Job drawing, mm, ordinate dimensions from the low corner. One solid piece. Coordinates: 2 decimals unless noted, no trailing zeros. Loops run counter-clockwise (first coordinate to the right, second up) from the corner with the lowest first, then second, coordinate; pieces in that order, holes last. Notation, with made-up numbers: M 82.25,2.5 L 129.25,2.5 A10 cw 129.25,14.5 Z; hole C 43.5,64.5 d5. An arc over 180 degrees is marked long. Answer as a JSON object with one key per item and string values. Group by question number.
1. Saw through at B-B on z = 116. Write the cut outline in (x, y), then the cut area to 3 significant figures.
2. Drill centre lines: L1, parallel to X at y = 6, z = 154; L2, parallel to X at y = 3.25, z = 77.5; L3, parallel to X at y = 2, z = 75. Where is each one in solid material? Low to high.
3. Saw through at A-A on z = 72. Write the cut outline in (x, y).
4. Saw through at C-C on x = 99. Write the cut outline in (y, z), then the cut area to 3 significant figures.
5. Drop a flat-ended pin along its axis: pin 1 Ø3.5 at (x, z) = (99, 154) entering from -Y. Give the stop position or say it passes through.
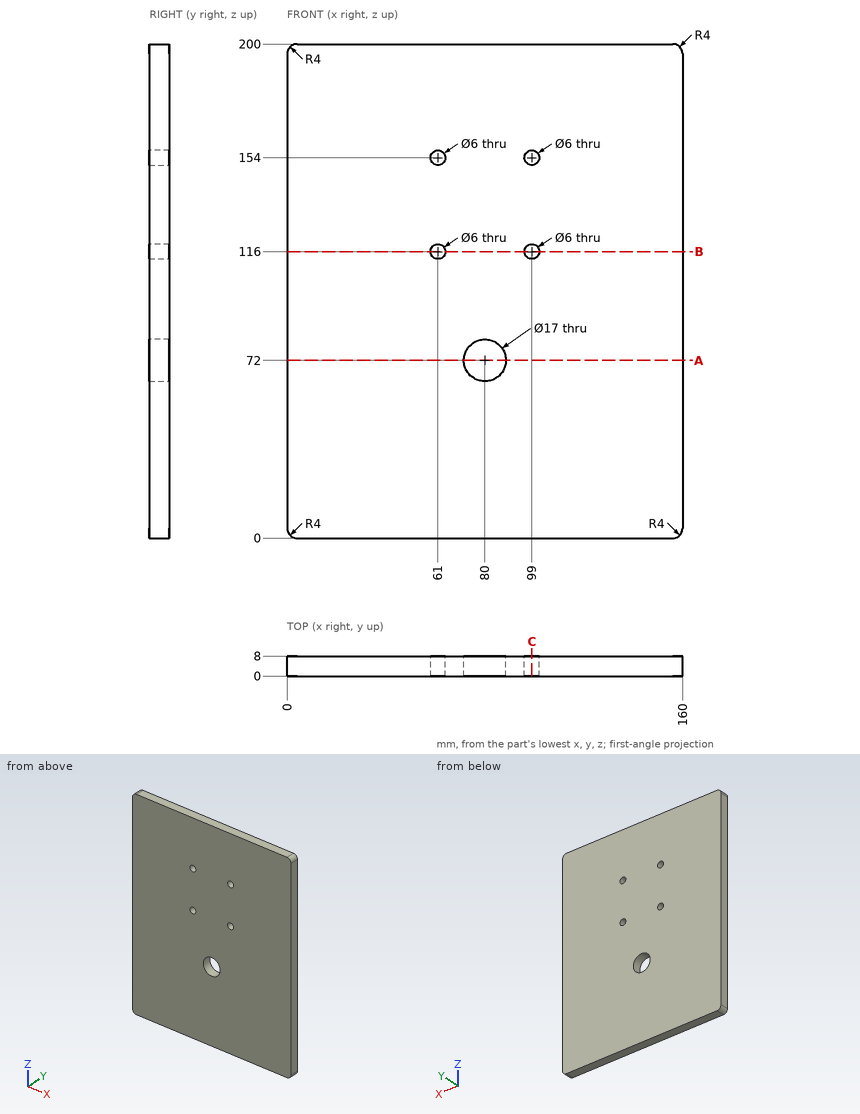
Outcome:
{
 "1": {"outline": "M 0,0 L 58,0 L 58,8 L 0,8 Z; M 64,0 L 96,0 L 96,8 L 64,8 Z; M 102,0 L 160,0 L 160,8 L 102,8 Z", "area": "1,180 mm²"},
 "2": {"L1": "x = 0 to 58, 64 to 96, 102 to 160", "L2": "x = 0 to 73.52, 86.48 to 160", "L3": "x = 0 to 72.05, 87.95 to 160"},
 "3": {"outline": "M 0,0 L 71.5,0 L 71.5,8 L 0,8 Z; M 88.5,0 L 160,0 L 160,8 L 88.5,8 Z"},
 "4": {"outline": "M 0,0 L 8,0 L 8,113 L 0,113 Z; M 0,119 L 8,119 L 8,151 L 0,151 Z; M 0,157 L 8,157 L 8,200 L 0,200 Z", "area": "1,500 mm²"},
 "5": {"pin 1": "passes through"}
}
